Autodesk Inventor part; units mm, degrees
ref_plane "YZ Plane" through (0, 0, 0) normal (1, 0, 0) x (0, 1, 0)
ref_plane "XZ Plane" through (0, 0, 0) normal (0, 1, 0) x (-1, 0, 0)
ref_plane "XY Plane" through (0, 0, 0) normal (0, 0, 1) x (1, 0, 0)
sketch "Sketch1" plane through (0, 0, 0) normal (0, 0, 1) x (1, 0, 0)
  line L0 (-98.425, 0) -> (98.425, 0)
  line L1 (98.425, 0) -> (98.425, 2.794)
  line L2 (98.425, 2.794) -> (-98.425, 2.794)
  line L3 (-98.425, 2.794) -> (-98.425, 0)
  line L4 (-88.9, 2.794) -> (-82.55, 60.6044)
  line L5 (-82.55, 60.6044) -> (82.55, 60.6044)
  line L6 (82.55, 60.6044) -> (88.9, 2.794)
  point P0 (0, 0)
  point P1 (0, 0)
  point P2 (0, 2.794)
  point P3 (0, 60.6044)
  dimension "d0" = 196.85
  dimension "d1" = 177.8
  dimension "d2" = 165.1
  dimension "d3" = 2.794
  dimension "d4" = 60.6044
extrude "Extrusion1" add sketch "Sketch1" along normal blind 101.6
sketch "Sketch2" plane through (-98.425, 0, 0) normal (0, -1, 0) x (1, 0, 0)
  line L0 (196.85, 101.6) -> (0, 101.6)
  line L1 (0, 0) -> (0, 101.6)
  line L2 (196.85, 0) -> (196.85, 101.6)
  line L3 (0, 83.4517) -> (5.207, 83.4517)
  line L4 (5.207, 83.4517) -> (5.207, 78.4733)
  line L5 (5.207, 78.4733) -> (0, 78.4733)
  line L6 (0, 78.4733) -> (0, 83.4517)
  circle A0 centre (5.207, 80.9625) radius 2.4892
  line L7 (0, 50.8) -> (196.85, 50.8)
  line L8 (98.425, 101.6) -> (98.425, 0)
  line L9 (0, 18.1483) -> (5.207, 18.1483)
  line L10 (5.207, 18.1483) -> (5.207, 23.1267)
  line L11 (5.207, 23.1267) -> (0, 23.1267)
  line L12 (0, 23.1267) -> (0, 18.1483)
  circle A1 centre (5.207, 20.6375) radius 2.4892
  line L13 (196.85, 83.4517) -> (191.643, 83.4517)
  line L14 (191.643, 83.4517) -> (191.643, 78.4733)
  line L15 (191.643, 78.4733) -> (196.85, 78.4733)
  line L16 (196.85, 78.4733) -> (196.85, 83.4517)
  circle A2 centre (191.643, 80.9625) radius 2.4892
  line L17 (196.85, 18.1483) -> (191.643, 18.1483)
  line L18 (191.643, 18.1483) -> (191.643, 23.1267)
  line L19 (191.643, 23.1267) -> (196.85, 23.1267)
  line L20 (196.85, 23.1267) -> (196.85, 18.1483)
  circle A3 centre (191.643, 20.6375) radius 2.4892
  dimension "d7" = 4.9784
  dimension "d8" = 5.207
  dimension "d9" = 30.1625
extrude "Extrusion2" cut sketch "Sketch2" against normal up to next contours L2 L17 A3 L19 | L11 A1 L9 L1 | L2 L15 A2 L13 | A2 L14 | L14 A2 | L3 A0 L5 L1 | A0 L4 | L4 A0 | A1 L10 | L10 A1 | A3 L18 | L18 A3
properties part number "supply-13.8"
For this review, take the finished solid that the model builds, in its own axes (mm). A direction names the side the tool comes from. Coordinates: 2 decimals unless noted, no trailing zeros. Write each loop counter-clockwise with the first axis right and the second up, starting at its lowest first coordinate (ties: lowest second). Pieces come first, ordered by that corner, then holes. Notation, with made-up numbers: (24, 63) -> (82, 63) arc R24 ccw to (82, 95) -> close; hole circle Ø6 at (-7, -37.5). An arc over 180 degrees is marked (long way). Write each question's results on one line, items separated by ' | '. Start each with the question number.
1) Wall thickness on L1, parallel to X at y = 57, z = 10; L2, parallel to X at y = 45, z = 15.5: over which ranges is each line inside the solid? List them lowest first. Write a range as [from, to].
2) Consider section C-C (x = 84.5). Write out the cut boundary in (y, z), plus the area to 3 significant figures.
3) Consider section A-A (z = 38). Write out the cut boundary in (x, y) (3 decimals), plus the area to 3 significant figures.
4) Insertion check: pin 1 (10 mm diameter, centred on y = 18.5, z = 13, fed in from +X); pin 2 (6 mm diameter, centred on y = 7.5, z = 43.5, fed in from +X); pin 3 (3 mm diameter, centred on x = 95, z = 55, fed in from +Y). Each pin has a flat end and moves straight along its axis. Give the tip position at first contact, or say it passes through.
5) Consider section B-B (y = 36.5). Write out the cut boundary in (x, z).
6) For faces 1 (the face through (-1, 0, 50)), 2 (the face through (-94, 2.794, 50)), 3 (the face through (94, 2.794, 50)), list the 3-axis set-ups (+Z, -Z, +X, -X, +Y, -Y) from which the entire face can be reached by the end or side of a thin tool; tool diameter is ignored.
Geometry says:
1) L1: [-82.95, 82.95] | L2: [-84.26, 84.26]
2) outline: (0, 0) -> (42.85, 0) -> (42.85, 101.6) -> (0, 101.6) -> close | area: 4,350 mm^2
3) outline: (-98.425, 0) -> (98.425, 0) -> (98.425, 2.794) -> (88.9, 2.794) -> (82.55, 60.604) -> (-82.55, 60.604) -> (-88.9, 2.794) -> (-98.425, 2.794) -> close | area: 10,500 mm^2
4) pin 1: x = 87.72 | pin 2: x = 88.71 | pin 3: y = 2.79
5) outline: (-85.2, 0) -> (85.2, 0) -> (85.2, 101.6) -> (-85.2, 101.6) -> close
6) face 1: +Z, -Z, +X, -X, -Y | face 2: +Z, -Z, -X, +Y | face 3: +Z, -Z, +X, +Y
